Autodesk Inventor part; units mm, degrees
ref_plane "Work Plane1" through (0.9879, 12, 10.2143) normal (0, 0, 1) x (1, 0, 0)
ref_plane "YZ Plane" through (0, 0, 0) normal (1, 0, 0) x (0, 1, 0)
ref_plane "XZ Plane" through (0, 0, 0) normal (0, 1, 0) x (-1, 0, 0)
sketch "Sketch1" plane through (0, 0, 0) normal (0, 1, 0) x (-1, 0, 0)
  line L0 (77.0121, 67.7143) -> (-2.9879, 67.7143)
  line L1 (-2.9879, 67.7143) -> (-2.9879, -12.2857)
  line L2 (-2.9879, -12.2857) -> (77.0121, -12.2857)
  line L3 (77.0121, -12.2857) -> (77.0121, 67.7143)
  point P0 (0, 0)
  dimension "d0" = 80
  dimension "d1" = 80
extrude "Extrusion1" add sketch "Sketch1" along normal blind 2
sketch "Sketch2" plane through (0, 2, 0) normal (0, 1, 0) x (1, 0, 0)
  line L0 (2.9879, -67.7143) -> (2.9879, 12.2857)
  line L1 (2.9879, 12.2857) -> (-77.0121, 12.2857)
  line L2 (-77.0121, 12.2857) -> (-77.0121, -67.7143)
  line L3 (-77.0121, -67.7143) -> (2.9879, -67.7143)
  line L4 (0.9879, -65.7143) -> (0.9879, 10.2857)
  line L5 (0.9879, 10.2857) -> (-75.0121, 10.2857)
  line L6 (-75.0121, 10.2857) -> (-75.0121, -65.7143)
  line L7 (-75.0121, -65.7143) -> (0.9879, -65.7143)
  point P0 (0, 0)
  dimension "d4" = 2
extrude "Extrusion2" add sketch "Sketch2" along normal blind 20
sketch "Sketch4" plane through (-77.0121, 0, 67.7143) normal (0, 0, 1) x (1, 0, 0)
  line L0 (2, 2) -> (2, 22)
  line L1 (78, 2) -> (78, 22)
  line L2 (2, 12) -> (78, 12)
  line L3 (78, 12) -> (78, 2)
  line L4 (78, 2) -> (2, 2)
  line L5 (2, 2) -> (2, 12)
  line L6 (2, 2) -> (78, 2)
  line L7 (78, 2) -> (78, 7)
  line L8 (78, 7) -> (2, 7)
  line L9 (2, 7) -> (2, 2)
  line L10 (78, 2) -> (62, 2)
  line L11 (62, 2) -> (2, 2)
  line L12 (2, 2) -> (78, 2)
  line L13 (2, 2) -> (62, 2)
  line L14 (2, 3.4) -> (78, 3.4)
  line L15 (2, 6.5) -> (78, 6.5)
  point P0 (77.0121, 0)
  point P1 (2, 3.4)
  dimension "d53" = 16
  dimension "d54" = 1.4
  dimension "d55" = 0.5
extrude "Extrusion4" cut sketch "Sketch4" against normal blind 20 contours L0 L15 L1 L14
sketch "Sketch5" plane through (0.9879, 2, -10.2857) normal (-1, 0, 0) x (0, 0, 1)
  line L0 (76, 0) -> (0, 0)
  line L1 (0, 0) -> (0, 20)
  circle A0 centre (10, 10) radius 9
  circle A1 centre (10, 10) radius 10
  circle A2 centre (10, 10) radius 10.5
  circle A3 centre (10, 10) radius 9.2
  line L2 (0, 20) -> (76, 20)
  line L3 (0, 10) -> (20.5, 10)
  line L4 (13.2016, 0) -> (16.2016, 0)
  line L5 (16.2016, 0) -> (16.2016, 1.5271)
  line L6 (10, 10) -> (10, 20)
  point P0 (10.2857, -2)
  point P1 (78, 0)
  point P2 (10, 0)
  point P3 (13.2016, 0)
  point P4 (13.2016, 20)
  point P5 (6.7984, 20)
  point P6 (0, 13.2016)
  point P7 (0.8, 10)
  point P8 (0, 10)
  point P9 (19.2, 10)
  point P10 (6.7984, 0)
  point P11 (0, 6.7984)
  point P12 (10, 19.2)
  dimension "d11" = 18
  dimension "d12" = 1
  dimension "d13" = 0.5
  dimension "d14" = 0.2
  dimension "d31" = 3
extrude "Extrusion5" add sketch "Sketch5" along normal blind 71 contours L0 A2 L5 | L0 A1 L3 A2 | L0 A2 L1 A1 | A1 L3 A3 | L0 L1 A2 | L1 A2 L2 A1 | A1 L6 A3 L3 | L1 L2 A2 picked at (0.4271, 11.4241)
sketch "Sketch10" plane through (0, 2, 0) normal (0, 1, 0) x (1, 0, 0)
  line L0 (-70.0121, -2.9159) -> (-70.0121, -10.2143)
  line L1 (-70.0121, 10.2857) -> (-75.0121, 10.2857)
  line L2 (-70.0121, -10.2143) -> (-71.5121, -10.2143)
  line L3 (-71.5121, -10.2143) -> (-71.5121, 10.2857)
  line L4 (-71.5121, 10.2857) -> (-70.0121, 10.2857)
  line L5 (-70.0121, 10.2857) -> (-70.0121, -10.2143)
  point P0 (0, 0)
  point P1 (-70.0121, -5.9159)
  dimension "d21" = 1.5
extrude "Extrusion8" add sketch "Sketch10" along normal up to surface (20 mm away)
sketch "Sketch11" plane through (-71.5121, 2, -10.2857) normal (-1, 0, 0) x (0, 0, 1)
  line L0 (20.5, 0) -> (0, 0)
  line L1 (20.5, 0) -> (20.5, 20)
  line L2 (0, 0) -> (0, 20)
  line L3 (20.5, 0) -> (20.5, 20)
  line L4 (0, 15) -> (20.5, 15)
  line L5 (6.75, 2) -> (13.75, 2)
  line L6 (13.75, 2) -> (13.75, 0)
  line L7 (0, 0) -> (0, 20)
  line L8 (20.5, 0) -> (0, 0)
  line L9 (6.75, 2) -> (6.75, 0)
  line L10 (20.5, 20) -> (0, 20)
  point P0 (10.2857, -2)
  point P1 (10.25, 2)
  point P2 (10.25, 15)
  dimension "d25" = 2
  dimension "d26" = 7
extrude "Extrusion9" cut sketch "Sketch11" along normal blind 4 and the other way blind 3 contours L0 L9 L5 L6
sketch "Sketch14" plane through (-70.0121, 2, 10.2143) normal (1, 0, 0) x (0, 0, -1)
  arc A0 (0, 10) -> (4.2984, 1.5271) centre (10.5, 10) ccw
  line L0 (0, 0) -> (0, 10)
  line L1 (4.2984, 0) -> (0, 0)
  line L2 (4.2984, 0) -> (4.2984, 1.5271)
  point P0 (10.2143, -2)
extrude "Extrusion11" cut sketch "Sketch14" against normal up to surface (5 mm away)
sketch "Sketch15" plane through (-70.0121, 12, 10.2143) normal (1, 0, 0) x (0, 0, -1)
  line L0 (4.2984, -10) -> (4.2984, -8.4729)
  line L1 (4.2984, -10) -> (4.2984, 5)
  line L2 (13.75, -8) -> (6.75, -8)
  line L3 (6.75, -8) -> (6.75, 5)
  line L4 (6.75, 5) -> (13.75, 5)
  line L5 (13.75, 5) -> (13.75, -8)
  point P0 (10.2143, -12)
  dimension "d35" = 15
extrude "Extrusion12" cut sketch "Sketch15" against normal blind 0.3
sketch "Sketch16" plane through (-70.0121, 12, 10.2143) normal (1, 0, 0) x (0, 0, -1)
  arc A0 (13.75, -8.6068) -> (10.5, 9.2) centre (10.5, 0) ccw
  arc A1 (0, 0) -> (4.2984, -8.4729) centre (10.5, 0) ccw
  circle A2 centre (10.5, 0) radius 10.5
  line L0 (10.5, 10) -> (0, 10)
  line L1 (0, 0) -> (0, 10)
  point P0 (10.2143, -12)
  point P1 (0, 0)
  point P2 (7.2984, 10)
extrude "Extrusion13" cut sketch "Sketch16" against normal up to surface (5 mm away) contours L1 L0 A2
sketch "Sketch17" plane through (-77.0121, 0, -12.2857) normal (-1, 0, 0) x (0, 0, 1)
  line L0 (0, 0) -> (0, 22)
  line L1 (25.5, 18) -> (43, 18)
  line L2 (43, 18) -> (43, 5.5)
  line L3 (43, 5.5) -> (25.5, 5.5)
  line L4 (25.5, 5.5) -> (25.5, 18)
  line L5 (0, 22) -> (80, 22)
  line L6 (43, 18) -> (43.7211, 18)
  line L7 (43.7211, 18) -> (43.7211, 5.5)
  line L8 (43.7211, 5.5) -> (43, 5.5)
  line L9 (25.5, 18) -> (25, 18)
  line L10 (25, 18) -> (25, 5.5)
  line L11 (25, 5.5) -> (25.5, 5.5)
  line L12 (25, 18) -> (25, 18.3)
  line L13 (25, 18.3) -> (43.7211, 18.3)
  line L14 (43.7211, 18.3) -> (43.7211, 18)
  point P0 (12.2857, 0)
  point P1 (20.2416, 9.7558)
  point P2 (0, 11)
  dimension "d46" = 12.5
  dimension "d47" = 17.5
  dimension "d50" = 4
  dimension "d51" = 0.5
  dimension "d52" = 0.3
extrude "Extrusion14" cut sketch "Sketch17" against normal blind 4
sketch "Sketch18" plane through (0.9879, 6.5, 65.7143) normal (-1, 0, 0) x (0, 0, 1)
  arc A0 (-66, 14.7) -> (-56.8, 5.5) centre (-66, 5.5) ccw
  point P0 (-65.7143, -6.5)
ref_plane "Work Plane1" through (0.9879, 12, 10.2143) normal (0, 0, 1) x (1, 0, 0)
sketch "Sketch19" plane through (0.9879, 12, 10.2143) normal (0, 0, 1) x (1, 0, 0)
  line L0 (-71, -8.401) -> (-71, 5)
  line L1 (-74.2989, 5) -> (0, 5)
  line L2 (0, 5) -> (0, 10)
  line L3 (0, 10) -> (-74.2989, 10)
  line L4 (-74.2989, 10) -> (-74.2989, 5)
  point P0 (-0.9879, -12)
extrude "Extrusion15" cut sketch "Sketch19" against normal up to surface (20.5 mm away)
properties part number "obudowa2"
Geometry: final body of the model. Coordinates: model frame, mm. A direction names the side the tool comes from. Coordinates: 2 decimals unless noted, no trailing zeros. Order: outer loops, then holes, each group sorted by start corner. A loop starts at its lowest first (then second) coordinate and runs counter-clockwise, first axis right, second up. Notation, with made-up numbers: (-10.75, 56.25) - (13.25, 56.25) arc R21 ccw to (13.25, 86.25) - close; hole circle Ø3 at (86.5, 33). An arc over 180 degrees is marked (long way). Return JSON: item names as keys, results as strings. Group by question number.
1. Cut plane D-D (y = 13.25). Output: boundary loops of the cut face in (x, z).
2. Cut plane A-A (z = 20). Output: boundary loops of the cut face in (x, y), plus the area to 3 significant figures.
3. Cut plane C-C (z = 62). Output: boundary loops of the cut face in (x, y).
4. Pull-direction query (X, two-part tool) for faces 1 (the face through (-77.012, 4, 27)), 2 (the face through (-38, 13, 67.714)), 3 (the face through (-75.012, 19, 28)); classes: pulls with the +X half, pulls with the -X half, needs draft (parallel to the pull), parting line crosses it, or undercut.
5. Material intervals for line 1 along X through (y, z) = (13.25, 42); line 2 along Z through (x, y) = (-7, 17.75); line 3 along X through (y, z) = (10.5, -1), sorted ascending. Write a range as [from, to].
6. Cut plane B-B (x = -20). Output: boundary loops of the cut face in (y, z), plus the area to 3 significant figures.
7. Set-up query: faces 4 (the face through (-34.02, 7.31, 9.11)), 5 (the face through (-76, 12, 31.435)), 6 (the face through (-38, 6.5, 67)), 7 (the face through (2.988, 11, 28)), 8 (the face through (-43.5, 17, -8.5)). Return all of +Z, -Z, +X, -X, +Y, -Y with unobstructed straight access to the full face (end or side cutting, diameter ignored); none if empty.
8. Pin query (flat end, axial travel): pin 1 (1 mm diameter, centred on x = -20, z = 38, fed in from +Y); pin 2 (0.6 mm diameter, centred on x = -31, z = 9.5, fed in from +Y). Return the tip coordinate at first contact, or that it passes through.
Resolved:
{
 "1": {"outline": "(-77.01, -12.29) - (2.99, -12.29) - (2.99, 67.71) - (-77.01, 67.71) - (-77.01, 31.44) - (-75.01, 31.44) - (-75.01, 65.71) - (0.99, 65.71) - (0.99, -9.4) - (-70.01, -9.4) - (-70.01, -3.54) - (-70.31, -3.54) - (-70.31, 3.46) - (-70.01, 3.46) - (-70.01, 10.14) - (-71.51, 10.14) - (-71.51, -10.29) - (-75.01, -10.29) - (-75.01, 12.71) - (-77.01, 12.71) - close"},
 "2": {"outline": "(-77.01, 0) - (2.99, 0) - (2.99, 22) - (0.99, 22) - (0.99, 2) - (-75.01, 2) - (-75.01, 5.5) - (-77.01, 5.5) - close; (-77.01, 18.3) - (-75.01, 18.3) - (-75.01, 22) - (-77.01, 22) - close", "area": "214 mm²"},
 "3": {"outline": "(-77.01, 0) - (2.99, 0) - (2.99, 22) - (0.99, 22) - (0.99, 2) - (-75.01, 2) - (-75.01, 22) - (-77.01, 22) - close"},
 "4": {"face 1": "pulls with the -X half", "face 2": "needs draft", "face 3": "undercut"},
 "5": {"line 1": "x = [-77.01, -75.01], [0.99, 2.99]", "line 2": "z = [-12.29, -10.29], [65.71, 67.71]", "line 3": "x = [-77.01, -75.01], [-71.51, -70.31], [0.99, 2.99]"},
 "6": {"outline": "(0, -12.29) - (22, -12.29) - (22, -10.29) - (17, -10.29) - (17, -8.01) arc R9.2 cw (long way) to (12, 8.91) - (12, 10.21) arc R10.5 ccw to (3.53, 5.92) - (2, 5.92) - (2, 65.71) - (3.4, 65.71) - (3.4, 67.71) - (0, 67.71) - close; (6.5, 65.71) - (22, 65.71) - (22, 67.71) - (6.5, 67.71) - close", "area": "295 mm²"},
 "7": {"face 4": "none", "face 5": "-X", "face 6": "+Z", "face 7": "+Z, -Z, +X, +Y, -Y", "face 8": "+Y"},
 "8": {"pin 1": "stops at y = 2", "pin 2": "stops at y = 12"}
}
